Read the model definition and answer for the solid it produces. Units are mm, in the model's axes. A direction names the side the tool comes from. Coordinates: 2 decimals unless noted, no trailing zeros. Write each loop counter-clockwise with the first axis right and the second up, starting at its lowest first coordinate (ties: lowest second). Pieces come first, ordered by that corner, then holes. Notation, with made-up numbers: (-16, 16.5) - (17, 16.5) arc R19 cw to (17, 45.5) - close; hole circle Ø10 at (-39.5, 28.25). An arc over 180 degrees is marked (long way). Use a Markdown table: item, result.
from build123d import *

# Parameters (mm, degrees)
SKETCH_2_W      = 0.8
SKETCH_2_H      = 5
EXTRUDE_1_DEPTH = 5


with BuildPart() as part:
    # Эскиз1 → Повернуть1 (revolve)
    with BuildSketch(Plane.XY):
        Polygon((0, 0), (8.25, 0), (8.25, 13), (9.5, 13), (6.5, 15), (6.5, 20), (0, 20), align=None)
    revolve(axis=Axis((0, -275.009579947, 0), (0, 1, 0)))

    # Эскиз2 → Бобышка-Вытянуть1 (add)
    with BuildSketch(Plane.XZ):
        with Locations((-4, 0)):
            Rectangle(SKETCH_2_W, SKETCH_2_H)
        with Locations((4, 0)):
            Rectangle(SKETCH_2_W, SKETCH_2_H)
    extrude(amount=EXTRUDE_1_DEPTH)


solid = part.part
(1) The mould has two halves that part along X. Classify faces 4 (the flat face through (4, -2, 2.5)), 5 (the cylindrical face through (7.62, 6.59, 3.16)), 6 (the flat face through (-3.6, -2, 0)): pulls with the +X half, pulls with the -X half, needs draft (parallel to the pull), parting line crosses it, or undercut.
Report:
| item | result |
|---|---|
| face 4 | needs draft |
| face 5 | parting line crosses it |
| face 6 | undercut |
(2) A cutting plane is placed at A-A, the plane z = 0. Write down the section's boundary in (x, y).
Report:
| item | result |
|---|---|
| outline | (-9.5, 13) - (-8.25, 13) - (-8.25, 0) - (-4.4, 0) - (-4.4, -5) - (-3.6, -5) - (-3.6, 0) - (3.6, 0) - (3.6, -5) - (4.4, -5) - (4.4, 0) - (8.25, 0) - (8.25, 13) - (9.5, 13) - (6.5, 15) - (6.5, 20) - (-6.5, 20) - (-6.5, 15) - close |
(3) Straight lines are drawn through the part: L1, parallel to Y at x = 2.5, z = 1.75; L2, parallel to X at y = 18.25, z = -2.75; L3, parallel to Y at x = -5.25, z = -6.5. For each, find the intervals that lie inside material, in ascending order.
Report:
| item | result |
|---|---|
| L1 | y = 0 to 20 |
| L2 | x = -5.89 to 5.89 |
| L3 | y = 13 to 13.76 |
(4) Each of these flat-tipped pins is pushed along its axis until it touches: P1, Ø1.5, axis at x = 1.5, y = 0.5, coming from the +Z side; P2, Ø2.5, axis at y = -2, z = 0.5, coming from the -X side; P3, Ø2, axis at x = -7.5, y = 0, coming from the -Z side. Where does it stop, or does it pass through?
Report:
| item | result |
|---|---|
| P1 | stops at z = 8.22 |
| P2 | stops at x = -4.4 |
| P3 | stops at z = -5.08 |
(5) For faces 1 (the flat face through (3, 13, -8)), 2 (the flat face through (3.6, -2, 0)), 3 (the flat face through (-4, -2, 2.5)), determine the directions among +Z, -Z, +X, -X, +Y, -Y from which every point of the face is accessible in a straight line to the end or side of a thin tool.
Report:
| item | result |
|---|---|
| face 1 | -Y |
| face 2 | +Z, -Z, -Y |
| face 3 | +Z, +X, -X, -Y |
(6) A cutting plane is placed at B-B, the plane x = 0. Write down the section's boundary in (y, z), and give its area (4 significant figures).
Report:
| item | result |
|---|---|
| outline | (0, -8.25) - (13, -8.25) - (13, -9.5) - (15, -6.5) - (20, -6.5) - (20, 6.5) - (15, 6.5) - (13, 9.5) - (13, 8.25) - (0, 8.25) - close |
| area | 311.5 mm² |
(7) A cutting plane is placed at C-C, the plane y = 12.5. Write down the section's boundary in (x, z), and give its area (3 significant figures).
Report:
| item | result |
|---|---|
| outline | circle Ø16.5 at (0, 0) |
| area | 214 mm² |
(8) A cutting plane is placed at D-D, the plane y = 15.5. Write down the section's boundary in (x, z).
Report:
| item | result |
|---|---|
| outline | circle Ø13 at (0, 0) |
